Could you check a few things on this model? Use its own coordinates, in mm. A direction names the side the tool comes from. Coordinates: 2 decimals unless noted, no trailing zeros. Write each loop counter-clockwise with the first axis right and the second up, starting at its lowest first coordinate (ties: lowest second). Pieces come first, ordered by that corner, then holes. Notation, with made-up numbers: M 68.5,-27 L 126.5,-27 A26 cw 126.5,-11 Z; hole C 21.25,70.25 d5. An arc over 180 degrees is marked long. Write item = value, one per line.
Autodesk Inventor part; units mm, degrees
ref_plane "YZ Plane" through (0, 0, 0) normal (1, 0, 0) x (0, 1, 0)
ref_plane "XZ Plane" through (0, 0, 0) normal (0, 1, 0) x (-1, 0, 0)
ref_plane "XY Plane" through (0, 0, 0) normal (0, 0, 1) x (1, 0, 0)
sketch "Sketch1" plane through (0, 0, 0) normal (1, 0, 0) x (0, 1, 0)
  line L0 (-5.1799, 0) -> (31.0792, 0) construction
  line L1 (0, -33.1988) -> (0, 40.25) construction
  line L2 (0, 0) -> (13, 9.7962) construction
  line L3 (0, 0) -> (13, -9.7962) construction
  line L4 (3.35, 2.6) -> (0.75, 2.6) construction
  line L5 (0.75, 2.6) -> (0.75, -2.6) construction
  line L6 (0.75, -2.6) -> (3.35, -2.6) construction
  line L7 (3.35, -2.6) -> (3.35, 2.6) construction
  line L8 (4.874, 11.4005) -> (4.874, -12.8161) construction
  line L9 (7.922, 11.2583) -> (7.922, -12.1988) construction
  circle A0 centre (6.398, 25.4) radius 3.175 construction
  line L10 (12.748, 29.7573) -> (12.748, -6.0773) construction
  line L11 (13, -8.155) -> (13, 15.6322) construction
  line L12 (12.748, 20.81) -> (8.422, 8.3886)
  line L13 (13, 11.8384) -> (4.874, 5.715) construction
  line L14 (12.9363, 20.81) -> (12.8744, 20.6322) construction
  line L15 (12.748, 20.81) -> (21.6933, 20.81) construction
  line L16 (12.9363, 20.81) -> (12.748, 20.81)
  line L17 (8.6773, 8.581) -> (8.422, 8.3886)
  line L18 (0, 3.81) -> (0, -3.81) construction
  line L19 (0, 3.81) -> (13, 13.6062) construction
  line L20 (13, 15.6322) -> (25.8994, 15.6322) construction
  line L21 (17.828, 20.81) -> (17.828, 20.6322)
  line L22 (17.828, 20.6322) -> (12.8744, 20.6322)
  line L23 (17.828, 20.81) -> (12.9363, 20.81)
  line L24 (12.8744, 20.6322) -> (8.6773, 8.581)
  line L25 (4.874, 5.715) -> (7.922, 8.763) construction
  line L26 (5, -22.7061) -> (5, -16.8713)
  line L27 (8.422, 8.3886) -> (8.422, 7.251) construction
  line L28 (8.422, 7.251) -> (3.35, 3.429) construction
  line L29 (6.398, 5.7258) -> (12.748, 13.6802) construction
  dimension "d0" = 37
  dimension "d1" = 13
  dimension "d2" = 2.6
  dimension "d3" = 5.2
  dimension "d4" = 0.75
  dimension "d5" = 1.524
  dimension "d6" = 3.048
  dimension "d7" = 6.35
  dimension "d8" = 1.524
  dimension "d9" = 25.4
  dimension "d10" = 3.175
  dimension "cone1_major_rad" = 20.81
  dimension "d13" = 0.5
  dimension "d15" = 5.715
  dimension "d17" = 0.1778
  dimension "d19" = 7.62
  dimension "d21" = 5.1778
  dimension "d22" = 0.1778
  dimension "ring_hieght" = 5.08
  dimension "cone1_minor_rad" = 8.3886
  dimension "cone1_height" = 4.326
  dimension "d26" = 45
  dimension "d27" = 5
  dimension "d29" = 2.286
  dimension "d30" = 7.251
  dimension "d31" = 13.6802
  dimension "cone2_minor_rad" = 5.7258
  dimension "d33" = 6.35
  dimension "d34" = 8.581
  dimension "cone2_hieght" = 2.024
revolve "Revolution1" add sketch "Sketch1" angle 360 about axis through (0, -10, 0) along (0, 1, 0)
sketch "Sketch2" plane through (0, 0, 0) normal (1, 0, 0) x (0, 1, 0)
  line L0 (8.6773, 8.581) -> (8.422, 8.3886)
  line L1 (0, 0) -> (13, 9.7962) construction
  line L2 (8.422, 8.3886) -> (8.422, 6.3464)
  line L3 (8.6773, 8.581) -> (8.6773, 6.5388)
  line L4 (8.422, 6.3464) -> (8.6773, 6.5388)
  line L5 (-5.1799, 0) -> (31.0792, 0) construction
revolve "Revolution2" [suppressed]
sketch "Sketch4" plane through (0, 0, 0) normal (1, 0, 0) x (0, 1, 0)
  line L0 (6.398, 5.7258) -> (12.748, 13.6802) construction
  line L1 (8.6773, 8.581) -> (6.398, 5.7258)
  line L2 (8.5383, 8.6919) -> (6.259, 5.8368)
  line L3 (6.398, 5.7258) -> (6.259, 5.8368)
  line L4 (8.6773, 8.581) -> (8.5383, 8.6919)
  line L5 (-5.1799, 0) -> (31.0792, 0) construction
  point P0 (0, 0)
  dimension "d36" = 0.1778
revolve "Revolution3" add sketch "Sketch4" angle 360 about axis through (0, -5.1799, 0) along (0, 1, 0)
equation "\"d8\" = 0.5 * d6"
equation "\"cone1_major_rad\" = 0.5 * main_aperture_diameter"
equation "\"d15\" = 0.5 * headplate_aperture_diameter"
equation "\"d19\" = fov_diameter"
equation "\"d21\" = 0.5 * EO_20x_diameter - 0.5 * E0_20x_front_aperture_diameter + d17"
equation "\"d22\" = d17"
equation "\"d36\" = d17"
equation "\"BendRadius\" = Thickness"
equation "\"BendReliefWidth\" = Thickness"
equation "\"BendReliefDepth\" = 0.5 * Thickness"
equation "\"CornerReliefSize\" = 4 * Thickness"
equation "\"MinimumRemnant\" = 2 * Thickness"
equation "\"TransitionRadius\" = BendRadius"
equation "\"JacobiRadiusSize\" = Thickness"
equation "\"GapSize\" = Thickness"
properties part number "objective_shield_2" material "Brass, Soft Yellow"
Item 1: If we mould it in two halves opening along Z, with no side actions, what happens to faces 3 (the face through (2.832, 8.784, 8.992)), 4 (the face through (-5.24, 6.54, 2.72))? For each: pulls with the +Z half, pulls with the -Z half, needs draft (parallel to the pull), parting line crosses it, or undercut.
Numbers:
face_3 = parting line crosses it
face_4 = undercut
Item 2: Imagine slicing it at C-C (y = 16.25). Write out the boundary of the cut face in (x, z), and give its area (3 significant figures).
Numbers:
outline = C 0,0 d41.62; hole C 0,0 d41.26
area = 23.1 mm²
Item 3: Imagine slicing it at A-A (x = 0). Write out the boundary of the cut face in (y, z), and give its area (3 significant figures).
Numbers:
outline = M 6.26,-5.84 L 8.52,-8.67 L 12.75,-20.81 L 17.83,-20.81 L 17.83,-20.63 L 12.87,-20.63 L 8.68,-8.58 L 6.4,-5.73 Z; M 6.26,5.84 L 6.4,5.73 L 8.68,8.58 L 12.87,20.63 L 17.83,20.63 L 17.83,20.81 L 12.75,20.81 L 8.52,8.67 Z
area = 7.63 mm²
Item 4: Imagine slicing it at D-D (y = 11.25). Write out the boundary of the cut face in (x, z), and give its area (3 significant figures).
Numbers:
outline = C 0,0 d33.02; hole C 0,0 d31.94
area = 55.2 mm²
Item 5: I'm going to push flat-ended pins straight in: P1, Ø1, axis at x = 1.5, z = 12, coming from the -Y side; P2, Ø1, axis at y = 14.5, z = -12.5, coming from the +X side; P3, Ø2, axis at x = 15.5, z = -16, coming from the +Y side. Where does each tip first touch, or does it pass through?
Numbers:
P1 = 9.54
P2 = 17
P3 = through
Item 6: For faces 1 (the face through (12.554, 15.317, -16.373)), 2 (the face through (1.806, 6.4, 5.736)), which set-ups out of +Z, -Z, +X, -X, +Y, -Y let a thin tool reach every point of the face, with its end or its side?
Numbers:
face_1 = +Y
face_2 = -Y
Item 7: If I drill on line 1 along X through (y, z) = (15, 0); line 2 along X through (y, z) = (13.25, -17.5); line 3 along Z through (x, y) = (-5, 14.25), over which ranges is the centre line in solid material (lowest first)?
Numbers:
line_1 = -20.81 to -20.63, 20.63 to 20.81
line_2 = -11.26 to -10.93, 10.93 to 11.26
line_3 = -20.2 to -20.02, 20.02 to 20.2
Item 8: Imagine slicing it at B-B (z = 0). Write out the boundary of the cut face in (x, y).
Numbers:
outline = M -20.81,12.75 L -8.67,8.52 L -5.84,6.26 L -5.73,6.4 L -8.58,8.68 L -20.63,12.87 L -20.63,17.83 L -20.81,17.83 Z; M 5.73,6.4 L 5.84,6.26 L 8.67,8.52 L 20.81,12.75 L 20.81,17.83 L 20.63,17.83 L 20.63,12.87 L 8.58,8.68 Z
